from build123d import *

# Parameters (mm, degrees)
SKETCH1_R           = 45
BOSS_EXTRUDE1_DEPTH = 50


with BuildPart() as part:
    # Sketch1 → Boss-Extrude1 (new body)
    with BuildSketch(Plane(origin=(0, 0, 0), x_dir=(1, 0, 0), z_dir=(0, 1, 0))):
        Circle(SKETCH1_R)
    extrude(amount=BOSS_EXTRUDE1_DEPTH)

    # Sketch2 → Cut-Revolve1 (revolve, cut)
    with BuildSketch(Plane(origin=(0, 0, 0), x_dir=(0, 0, -1), z_dir=(1, 0, 0))):
        Polygon((0, 50), (0, 0), (-40, 0), (-40, 10), (-37, 10), (-6, 41), (-6, 50), align=None)
    revolve(axis=Axis((0, 50, 0), (0, -1, 0)), mode=Mode.SUBTRACT)


solid = part.part
The listing builds one solid part. Answer for the finished solid, in the listing's coordinates (mm). A direction names the side the tool comes from. Coordinates: 2 decimals unless noted, no trailing zeros. Loops run counter-clockwise (first coordinate to the right, second up) from the corner with the lowest first, then second, coordinate; pieces in that order, holes last.
1) Find section C-C on y = 13.5. Write down the section's boundary in (x, z).
2) A tool of negligible diameter and unlimited length cuts with its end or side. For faces 4 (the face through (39.05, 5.07, -8.67)), 5 (the face through (0, 46, -6)), from which of +Z, -Z, +X, -X, +Y, -Y can it reach the whole face along a straight path? Write none if from no direction.
3) Find section B-B on z = 0. Write down the section's boundary in (x, y).
4) Find section A-A on x = 0. Write down the section's boundary in (y, z).
5) Find section D-D on y = 35. Write down the section's boundary in (x, z).
6) Determine the mould class of faces 1 (the face through (-1, 50, 9)), 2 (the face through (20.765, 24.65, 39.923)), 3 (the face through (35.4, 10, 11.7)) for opening direction X: pulls with the +X half, pulls with the -X half, needs draft (parallel to the pull), parting line crosses it, or undercut.
7) Flat-ended cylindrical pins translate along their axes: pin 1 Ø12 at (x, y) = (30, 31.5) entering from +Z; pin 2 Ø3 at (y, z) = (42.5, -17) entering from +X; pin 3 Ø4 at (y, z) = (9.5, 14.5) entering from -X. Find the tip coordinate at first contact, or state that the pin passes through.
8) Find the intervals of material crossed by L1, parallel to Z at x = 0, y = 5.75; L2, parallel to X at y = 46.25, z = 0, in increasing order.
Values:
1. outline: circle Ø90 at (0, 0); hole circle Ø67 at (0, 0)
2. face 4: -Y
2. face 5: +Y, -Y
3. outline: (-45, 0) - (-40, 0) - (-40, 10) - (-37, 10) - (-6, 41) - (-6, 50) - (-45, 50) - close; (6, 41) - (37, 10) - (40, 10) - (40, 0) - (45, 0) - (45, 50) - (6, 50) - close
4. outline: (0, -45) - (50, -45) - (50, -6) - (41, -6) - (10, -37) - (10, -40) - (0, -40) - close; (0, 40) - (10, 40) - (10, 37) - (41, 6) - (50, 6) - (50, 45) - (0, 45) - close
5. outline: circle Ø90 at (0, 0); hole circle Ø24 at (0, 0)
6. face 1: needs draft
6. face 2: parting line crosses it
6. face 3: undercut
7. pin 1: stops at z = 38.07
7. pin 2: stops at x = 42.25
7. pin 3: stops at x = -43.23
8. L1: z = -45 to -40, 40 to 45
8. L2: x = -45 to -6, 6 to 45
